Study the drawing (mm; zero at the part's minimum x, y, z) and answer. A direction names the side the tool comes from. Round coordinates to 2 decimals unless told otherwise and drop trailing zeros. Loops run counter-clockwise (first coordinate to the right, second up) from the corner with the lowest first, then second, coordinate; pieces in that order, holes last. Notation, with made-up numbers: (83.5, -36.5) - (117.5, -36.5) arc R6 ccw to (117.5, -26.5) - close; hole circle Ø1 at (63.5, 53.5). An arc over 180 degrees is marked (long way). One line per item, written item: value.
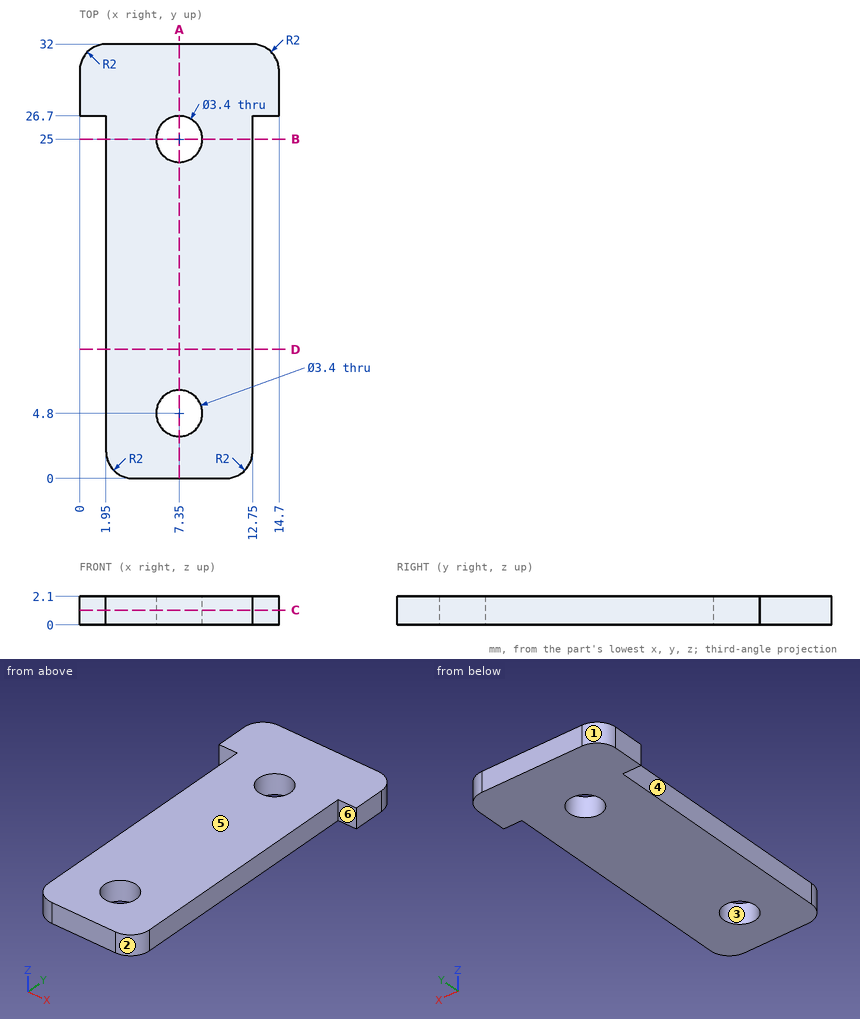
1) A cutting plane is placed at B-B on y = 25. Give the vertices of the cut face in (x, z).
Final values:
outline: (1.95, 0) - (5.65, 0) - (5.65, 2.1) - (1.95, 2.1) - close; (9.05, 0) - (12.75, 0) - (12.75, 2.1) - (9.05, 2.1) - close
2) A cutting plane is placed at C-C on z = 1.1. Give the vertices of the cut face in (x, y).
Final values:
outline: (0, 26.7) - (1.95, 26.7) - (1.95, 2) arc R2 ccw to (3.95, 0) - (10.75, 0) arc R2 ccw to (12.75, 2) - (12.75, 26.7) - (14.7, 26.7) - (14.7, 30) arc R2 ccw to (12.7, 32) - (2, 32) arc R2 ccw to (0, 30) - close; hole circle Ø3.4 at (7.35, 4.8); hole circle Ø3.4 at (7.35, 25)
3) A cutting plane is placed at D-D on y = 9.5. Give the vertices of the cut face in (x, z).
Final values:
outline: (1.95, 0) - (12.75, 0) - (12.75, 2.1) - (1.95, 2.1) - close
4) Each of these flat-tipped pins is pushed along its axis until it touches: pin 1 Ø1 at (y, z) = (18, 1) entering from -X; pin 2 Ø0.6 at (y, z) = (17, 1.5) entering from +X; pin 3 Ø0.6 at (x, z) = (14, 1) entering from -Y. Where does it stop, or does it pass through?
Final values:
pin 1: x = 1.95
pin 2: x = 12.75
pin 3: y = 26.7
5) For a pull along Y with two mould halves and no side action, classify the marked faces 1, 2 and 3 as released by +Y, released by -Y, zero draft, split by the parting line, or undercut.
Final values:
face 1: released by +Y
face 2: released by -Y
face 3: undercut
6) Consider L1, parallel to Y at x = 7.35, z = 0.95; L2, parallel to Y at x = 8, z = 1.85; L3, parallel to X at y = 23.5, z = 1.05. Determine where each line is inside the solid, lowest interval first.
Final values:
L1: 0 to 3.1, 6.5 to 23.3, 26.7 to 32
L2: 0 to 3.23, 6.37 to 23.43, 26.57 to 32
L3: 1.95 to 6.55, 8.15 to 12.75
7) For the marked faces 4, 5 and 6, determine the directions among +Z, -Z, +X, -X, +Y, -Y from which every point of the face is accessible in a straight line to the end or side of a thin tool.
Final values:
face 4: +Z, -Z, -X, -Y
face 5: +Z, +X, -X, +Y, -Y
face 6: +Z, -Z, +X, -Y
8) A cutting plane is placed at A-A on x = 7.35. Give the vertices of the cut face in (y, z).
Final values:
outline: (0, 0) - (3.1, 0) - (3.1, 2.1) - (0, 2.1) - close; (6.5, 0) - (23.3, 0) - (23.3, 2.1) - (6.5, 2.1) - close; (26.7, 0) - (32, 0) - (32, 2.1) - (26.7, 2.1) - close
